Input: dimensioned drawing with shaded views. Units: mm. Origin: part minimum x, y, z. A direction names the side the tool comes from. Coordinates: 2 decimals unless noted, no trailing zeros. Loops run counter-clockwise (first coordinate to the right, second up) from the corner with the lowest first, then second, coordinate; pieces in that order, holes last.
Item 1: Section query D-D, the plane y = 18. Return the cut outline in (x, z).
Item 2: Section query C-C, the plane z = 6. Return the cut outline in (x, y) (1 decimal), then the cut area to 3 significant figures.
Item 3: Pin query (flat end, axial travel): pin 1 Ø3 at (y, z) = (20.5, 26) entering from -X; pin 2 Ø8 at (x, z) = (20.5, 19) entering from -Y; pin 3 Ø4 at (x, y) = (94, 7) entering from -Z. Return the tip coordinate at first contact, or that it passes through.
Item 4: Reachability of the marked faces 1 and 2 from +Z, -Z, +X, -X, +Y, -Y: full face, straight path, thin tool, end or side. Return the list, or none.
Item 5: Section query B-B, the plane y = 36.5. Return the cut outline in (x, z).
Item 6: Line query: probe 1 along X at (y, z) = (10.5, 21.5); probe 2 along Y at (x, z) = (90, 15.5) (1 decimal); probe 3 along Z at (x, y) = (31, 35). Output: solid intervals per line, ascending.
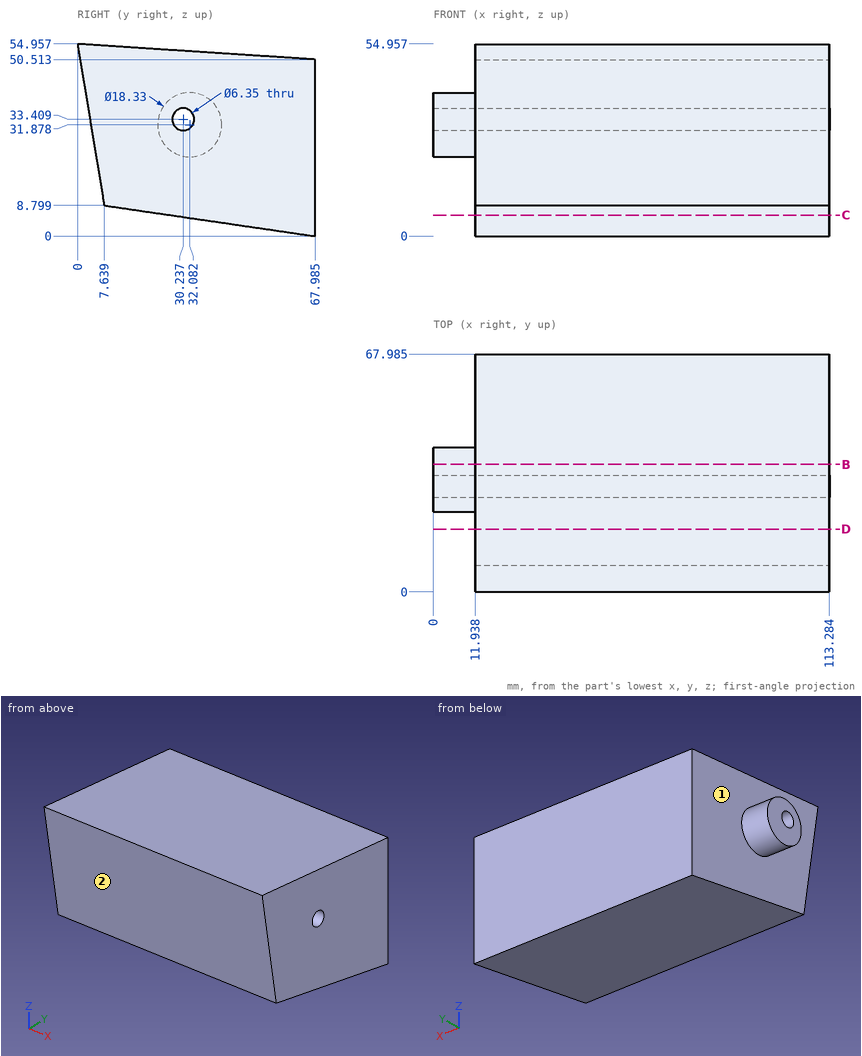
Verdict:
1. outline: (11.94, 7.29) - (113.28, 7.29) - (113.28, 53.78) - (11.94, 53.78) - close
2. outline: (11.9, 26.8) - (113.3, 26.8) - (113.3, 68) - (11.9, 68) - close
2. area: 4,170 mm2
3. pin 1: stops at x = 11.94
3. pin 2: stops at y = 5.29
3. pin 3: stops at z = 8.6
4. face 1: -X
4. face 2: -Z, +X, -X, -Y
5. outline: (0, 23.85) - (11.94, 23.85) - (11.94, 4.59) - (113.28, 4.59) - (113.28, 52.57) - (11.94, 52.57) - (11.94, 39.91) - (0, 39.91) - close
6. probe 1: x = 11.94 to 113.28
6. probe 2: y = 6.5 to 68
6. probe 3: z = 4.81 to 52.67
